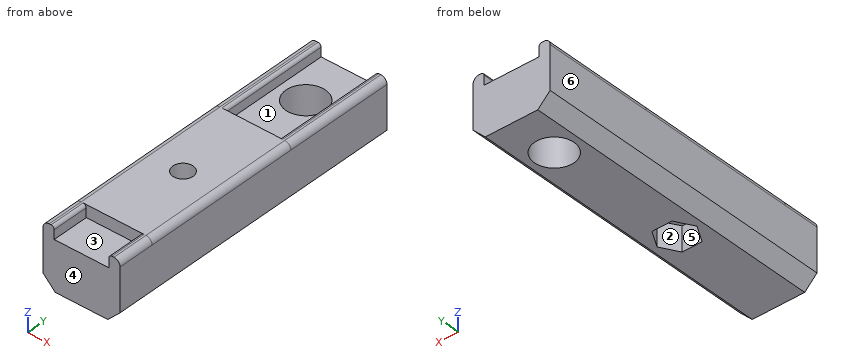
from build123d import *

# Parameters (mm, degrees)
BOSS_EXTRUDE1_DEPTH = 50
CUT_EXTRUDE2_DEPTH  = 53.511927217
FILLET1_R           = 0.5
SKETCH4_R           = 3.225
SKETCH4_R_2         = 1.65
CUT_EXTRUDE3_DEPTH  = 53.511927217
BOSS_EXTRUDE2_REACH = 54.024
SKETCH5_W           = 12.55
SKETCH5_H           = 26
SKETCH5_R           = 1.65
FILLET2_R           = 1
CUT_EXTRUDE4_DEPTH  = 4
BOSS_EXTRUDE3_DEPTH = 18
SKETCH8_R           = 3.225
CUT_EXTRUDE5_DEPTH  = 53.024056935
BOSS_EXTRUDE4_DEPTH = 6


with BuildPart() as part:
    # Sketch1 → Boss-Extrude1 (new body)
    with BuildSketch(Plane(origin=(0, 0, 0), x_dir=(1, 0, 0), z_dir=(0, 1, 0))):
        with BuildLine():
            Line((0, 8), (2, 10))
            Line((2, 10), (10.55, 10))
            Line((10.55, 10), (12.55, 8))
            Line((12.55, 8), (12.55, 1))
            ThreePointArc((12.55, 1), (12.257106781, 0.292893219), (11.55, 0))
            Line((11.55, 0), (1, 0))
            ThreePointArc((1, 0), (0.292893219, 0.292893219), (0, 1))
            Line((0, 1), (0, 8))
        make_face()
    extrude(amount=BOSS_EXTRUDE1_DEPTH)

    # Sketch3 → Cut-Extrude2 (cut, through all)
    with BuildSketch(Plane.XZ):
        Polygon((1.825, 0), (1.825, -2), (2.825, -3), (9.725, -3), (10.725, -2), (10.725, 0), align=None)
    extrude(amount=-CUT_EXTRUDE2_DEPTH, mode=Mode.SUBTRACT)

    # Fillet1
    fillet1_edges = [part.edges().sort_by_distance(p)[0] for p in [
        (1.825, 25, 0),
        (10.725, 25, 0),
    ]]
    fillet(fillet1_edges, radius=FILLET1_R)

    # Sketch4 → Cut-Extrude3 (cut, through all)
    with BuildSketch(Plane(origin=(0, 0, -10), x_dir=(-1, 0, 0), z_dir=(0, 0, -1))):
        with Locations((-6.275, 42)):
            Circle(SKETCH4_R)
        with Locations((-6.275, 19)):
            Circle(SKETCH4_R_2)
    extrude(amount=-CUT_EXTRUDE3_DEPTH, mode=Mode.SUBTRACT)

    # Boss-Extrude2: up to this face of the body (flat: up to its plane)
    boss_extrude2_end = Plane(part.part.faces().sort_by_distance((1.1625, 25, 0))[0])
    # Sketch5 → Boss-Extrude2 (add, up to the picked face)
    with BuildSketch(Plane.XY.offset(-3), mode=Mode.PRIVATE) as boss_extrude2_sk1:
        with Locations((6.275, 19)):
            Rectangle(SKETCH5_W, SKETCH5_H)
        with Locations(Location((6.275, 19, 0), (0, 0, 180))):
            Circle(SKETCH5_R, mode=Mode.SUBTRACT)
    boss_extrude2_tool1 = split(extrude(boss_extrude2_sk1.sketch, amount=BOSS_EXTRUDE2_REACH, mode=Mode.PRIVATE), bisect_by=boss_extrude2_end, keep=Keep.BOTH, mode=Mode.PRIVATE)
    add(boss_extrude2_tool1.solids().sort_by(Axis((6.275, 6.288704, -3), (0, 0, 1)))[0])

    # Fillet2
    fillet2_edges = [part.edges().sort_by_distance(p)[0] for p in [
        (12.55, 19, 0),
        (0, 19, 0),
    ]]
    fillet(fillet2_edges, radius=FILLET2_R)

    # Sketch6 → Cut-Extrude4 (cut)
    with BuildSketch(Plane(origin=(0, 0, -10), x_dir=(-1, 0, 0), z_dir=(0, 0, -1))):
        Polygon((-3.012970979, 19), (-4.64398549, 21.825), (-7.90601451, 21.825), (-9.537029021, 19), (-7.90601451, 16.175), (-4.64398549, 16.175), align=None)
    extrude(amount=-CUT_EXTRUDE4_DEPTH, mode=Mode.SUBTRACT)

    # Sketch7 → Boss-Extrude3 (add)
    with BuildSketch(Plane(origin=(0, 32, 0), x_dir=(1, 0, 0), z_dir=(0, 1, 0))):
        Polygon((1.825, 2), (10.725, 2), (9.725, 3), (2.825, 3), align=None)
    extrude(amount=BOSS_EXTRUDE3_DEPTH)

    # Sketch8 → Cut-Extrude5 (cut, through all)
    with BuildSketch(Plane(origin=(0, 0, -3), x_dir=(-1, 0, 0), z_dir=(0, 0, -1))):
        with Locations((-6.275, 42)):
            Circle(SKETCH8_R)
    extrude(amount=-CUT_EXTRUDE5_DEPTH, mode=Mode.SUBTRACT)

    # Sketch9 → Boss-Extrude4 (add)
    with BuildSketch(Plane.XZ.offset(-6)):
        Polygon((1.825, -2), (10.725, -2), (9.725, -3), (2.825, -3), align=None)
    extrude(amount=BOSS_EXTRUDE4_DEPTH)


solid = part.part
Read the model definition and answer for the solid it produces. Units are mm, in the model's axes. Face numbers are marked on the shaded views. A direction names the side the tool comes from. Coordinates: 2 decimals unless noted, no trailing zeros. Loops run counter-clockwise (first coordinate to the right, second up) from the corner with the lowest first, then second, coordinate; pieces in that order, holes last.
Q1. Each of these flat-tipped pins is pushed along its axis until it touches: pin 1 Ø3 at (x, y) = (6.5, 2) entering from +Z; pin 2 Ø1.7 at (x, y) = (7, 19.5) entering from -Z; pin 3 Ø0.6 at (x, z) = (8.5, -1) entering from -Y. Where does it stop, or does it pass through?
Q2. The part is cut by section C-C on y = 47. Write down the section's boundary in (x, z) (3 decimals).
Q3. Consider probe 1 along Y at (x, z) = (6.25, -3.5); probe 2 along X at (y, z) = (33, -1.5) (3 decimals); probe 3 along Z at (x, y) = (2, 43.5). Determine where each line is inside the solid, lowest interval first.
Q4. The part is cut by section A-A on z = -7.5. Write down the section's boundary in (x, y) (3 decimals), and give its area (3 significant figures).
Q5. Which of the six approach directions +Z, -Z, +X, -X, +Y, -Y give full straight-line access (tool end or side, diameter ignored) to the marked faces 1, 2 and 3?
Q6. The part is cut by section D-D on x = 8.5. Write down the section's boundary in (y, z), and give its area (3 significant figures).
Q7. The part is cut by section B-B on y = 42. Write down the section's boundary in (x, z) (3 decimals).
Q8. The mould has two halves that part along Y. Classify the marked faces 4, 5 and 6: +Y half, -Y half, draft (parallel to the pull), parting line (faces both ways), or undercut.
Results below:
1. pin 1: stops at z = -2
1. pin 2: stops at z = -6
1. pin 3: stops at y = 6
2. outline: (0, -8) - (2, -10) - (10.55, -10) - (12.55, -8) - (12.55, -1) arc R1 ccw to (11.55, 0) - (11.225, 0) arc R0.5 ccw to (10.725, -0.5) - (10.725, -2) - (1.825, -2) - (1.825, -0.5) arc R0.5 ccw to (1.325, 0) - (1, 0) arc R1 ccw to (0, -1) - close
3. probe 1: y = 0 to 17.35, 20.65 to 38.78, 45.22 to 50
3. probe 2: x = 0 to 1.825, 10.725 to 12.55
3. probe 3: z = -10 to -2
4. outline: (0, 0) - (12.55, 0) - (12.55, 50) - (0, 50) - close; hole (3.013, 19) - (4.644, 16.175) - (7.906, 16.175) - (9.537, 19) - (7.906, 21.825) - (4.644, 21.825) - close; hole circle Ø6.45 at (6.275, 42)
4. area: 567 mm2
5. face 1: +Z, +Y
5. face 2: -Z
5. face 3: +Z, -Y
6. outline: (0, -10) - (17.2, -10) - (17.2, -6) - (20.8, -6) - (20.8, -10) - (39.67, -10) - (39.67, -2) - (32, -2) - (32, 0) - (6, 0) - (6, -2) - (0, -2) - close; (44.33, -10) - (50, -10) - (50, -2) - (44.33, -2) - close
6. area: 400 mm2
7. outline: (0, -8) - (2, -10) - (3.05, -10) - (3.05, -2) - (1.825, -2) - (1.825, -0.5) arc R0.5 ccw to (1.325, 0) - (1, 0) arc R1 ccw to (0, -1) - close; (9.5, -10) - (10.55, -10) - (12.55, -8) - (12.55, -1) arc R1 ccw to (11.55, 0) - (11.225, 0) arc R0.5 ccw to (10.725, -0.5) - (10.725, -2) - (9.5, -2) - close
8. face 4: -Y half
8. face 5: undercut
8. face 6: draft
